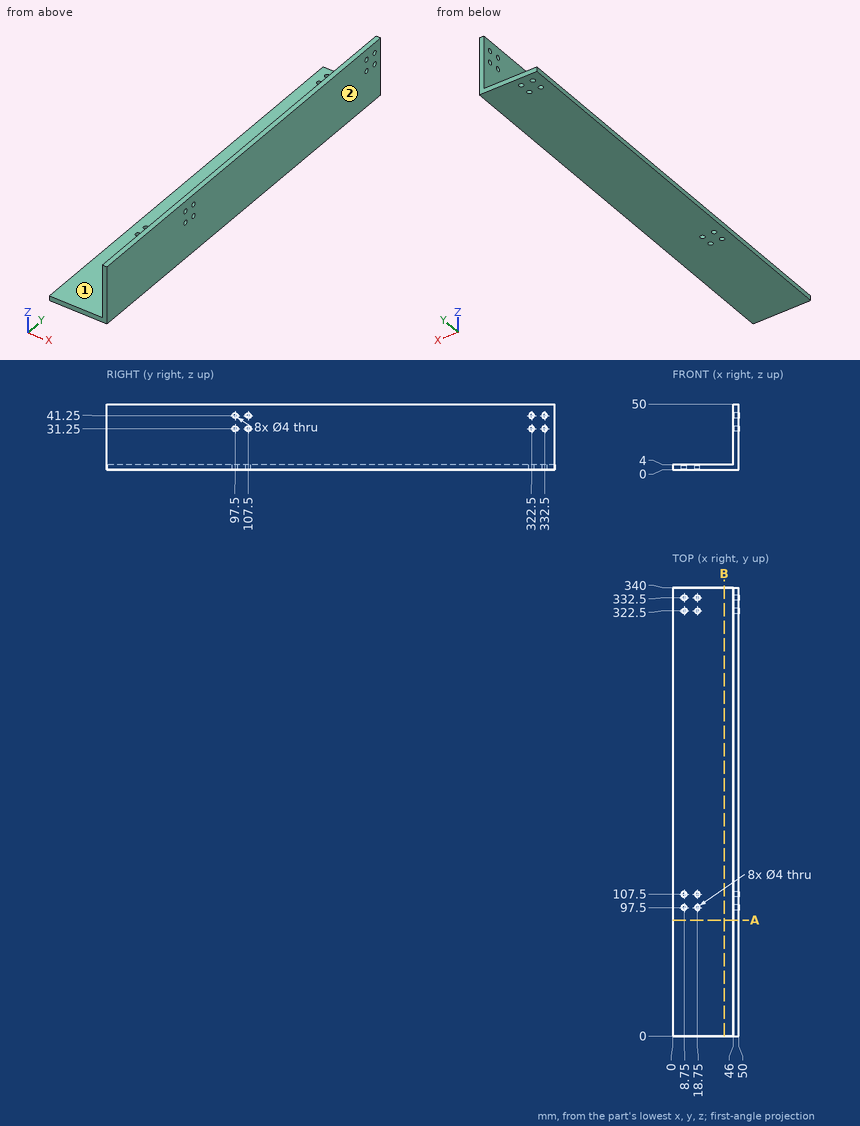
Study the drawing (mm; zero at the part's minimum x, y, z) and answer. A direction names the side the tool comes from. Coordinates: 2 decimals unless noted, no trailing zeros. Write each loop counter-clockwise with the first axis right and the second up, starting at its lowest first coordinate (ties: lowest second). Pieces come first, ordered by that corner, then holes. Notation, with made-up numbers: (66, -11.75) - (103, -11.75) arc R22 cw to (103, 7.25) - close; hole circle Ø5 at (36, -35). An arc over 180 degrees is marked (long way). Answer as a JSON object with one key per item and string values.
Q1. Find section A-A (y = 88). Write down the section's boundary in (x, z), plus the area to 3 significant figures.
Results list:
{"outline": "(0, 0) - (50, 0) - (50, 50) - (46, 50) - (46, 4) - (0, 4) - close", "area": "384 mm^2"}
Q2. Which of the six approach directions +Z, -Z, +X, -X, +Y, -Y give full straight-line access (tool end or side, diameter ignored) to the marked faces 1 and 2?
Results list:
{"face 1": "+Z, -X, +Y, -Y", "face 2": "+Z, -Z, +X, +Y, -Y"}
Q3. Consider L1, parallel to Z at x = 47.9, y = 107.5; L2, parallel to Y at x = 8.75, z = 0.8; L3, parallel to X at y = 322.5, z = 2.2. Determine where each line is inside the solid, lowest interval first. Write a range as from..to.
Results list:
{"L1": "z = 0..29.25, 33.25..39.25, 43.25..50", "L2": "y = 0..95.5, 99.5..105.5, 109.5..320.5, 324.5..330.5, 334.5..340", "L3": "x = 0..6.75, 10.75..16.75, 20.75..50"}
Q4. Find section B-B (x = 39). Write down the section's boundary in (y, z), plus the area to 3 significant figures.
Results list:
{"outline": "(0, 0) - (340, 0) - (340, 4) - (0, 4) - close", "area": "1,360 mm^2"}
Q5. Given pin 1 Ø2 at (y, z) = (155, 26.5) entering from -X; pin 2 Ø3.5 at (x, y) = (8.75, 322.5) entering from +Z; pin 3 Ø2 at (x, y) = (8.5, 254) entering from +Z, each flat-ended and moving along its own axis, determine where each tip first touches the part or whether it passes through.
Results list:
{"pin 1": "stops at x = 46", "pin 2": "passes through", "pin 3": "stops at z = 4"}
